from build123d import *

# Parameters (mm, degrees)
F0_R     = 8
F0_R_2   = 7
F1_DEPTH = 8.15
F2_DEPTH = 10
F3_DEPTH = 9
F5_W     = 115
F5_H     = 65
F6_DEPTH = 0.5
F8_DEPTH = 20
F11_R    = 1.5


# Not quite as in the source:
# - a fillet or chamfer that OpenCascade refuses, or shapes differently, is made with other operations: its cross-section is extruded or revolved along the edge and cut away or added


with BuildPart() as f1:
    # F0 (on Top) → F1 (new body)
    with BuildSketch(Plane.XY):
        with BuildLine():
            Line((-67.5, -39), (67.5, -39))
            ThreePointArc((67.5, -39), (71.7426406871, -37.2426406871), (73.5, -33))
            Line((73.5, -33), (73.5, 33))
            ThreePointArc((73.5, 33), (71.7426406871, 37.2426406871), (67.5, 39))
            Line((67.5, 39), (-67.5, 39))
            ThreePointArc((-67.5, 39), (-71.7426406871, 37.2426406871), (-73.5, 33))
            Line((-73.5, 33), (-73.5, -33))
            ThreePointArc((-73.5, -33), (-71.7426406871, -37.2426406871), (-67.5, -39))
        make_face()
        with Locations((-53.5, 0)):
            Circle(F0_R, mode=Mode.SUBTRACT)
        with Locations((-30.5, 0)):
            Circle(F0_R_2, mode=Mode.SUBTRACT)
        with Locations((-53.5, 0)):
            Circle(F0_R)
        with Locations((-30.5, 0)):
            Circle(F0_R_2)
    extrude(amount=F1_DEPTH)

    # F0 (on Top) → F2 (join)
    with BuildSketch(Plane.XY):
        with Locations((-53.5, 0)):
            Circle(F0_R)
    extrude(amount=F2_DEPTH)

    # F0 (on Top) → F3 (join)
    with BuildSketch(Plane.XY):
        with Locations((-30.5, 0)):
            Circle(F0_R_2)
    extrude(amount=F3_DEPTH)

    # F4: fillet of radius 4 on 1 edges, made by hand

    # F4_s1 → F4_t2 (revolve)
    with BuildSketch(Plane.XZ):
        with BuildLine():
            ThreePointArc((-42.1269450049, 8.15), (-44.0504834111, 8.6428644167), (-45.5, 10))
            Line((-45.5, 10), (-45.5, 8.15))
            Line((-45.5, 8.15), (-42.1269450049, 8.15))
        make_face()
    revolve(axis=Axis((-53.5, 0, 8.15), (0, 0, -1)))

    # F5 (on Top) → F6 (cut)
    with BuildSketch(Plane.XY):
        Rectangle(F5_W, F5_H)
    extrude(amount=F6_DEPTH, mode=Mode.SUBTRACT)

    # F7 (on face) → F8 (join)
    with BuildSketch(Plane.YZ.offset(73.5)):
        with BuildLine():
            ThreePointArc((7.4520160146, 3), (9.4520160146, 5), (7.4520160146, 7))
            Line((7.4520160146, 7), (-6.5479839854, 7))
            ThreePointArc((-6.5479839854, 7), (-8.5479839854, 5), (-6.5479839854, 3))
            Line((-6.5479839854, 3), (7.4520160146, 3))
        make_face()
        with BuildLine():
            ThreePointArc((-1.5, 5), (0, 6.5), (1.5, 5))
            ThreePointArc((1.5, 5), (0, 3.5), (-1.5, 5))
        make_face(mode=Mode.SUBTRACT)
        with BuildLine():
            Line((-1.5, 5), (1.5, 5))
            ThreePointArc((1.5, 5), (0, 6.5), (-1.5, 5))
        make_face()
        with BuildLine():
            ThreePointArc((-1.5, 5), (0, 3.5), (1.5, 5))
            Line((1.5, 5), (-1.5, 5))
        make_face()
    extrude(amount=F8_DEPTH)

    # F12: sweep along a path in F10
    with BuildLine(Plane(origin=(0, 0, 5), x_dir=(1, 0, 0), z_dir=(0, 0, -1))) as f12_path:
        ThreePointArc((93.5, 0), (108.8125986956, 5.7360841116), (116.8597106736, 19.970631121))
    # F11 (on face) → F12 (sweep)
    with BuildSketch(Plane.YZ.offset(93.5)):
        with Locations((0, 5)):
            Circle(F11_R)
    sweep(path=f12_path.line)


solid = f1.part
Geometry check sheet. Reference: the model listing, model coordinates, mm. A direction names the side the tool comes from. Round coordinates to 2 decimals unless told otherwise and drop trailing zeros. Loops run counter-clockwise (first coordinate to the right, second up) from the corner with the lowest first, then second, coordinate; pieces in that order, holes last. Notation, with made-up numbers: (81, -40) - (104, -40) arc R9 cw to (104, -23) - close; hole circle Ø9 at (-19, 9). An arc over 180 degrees is marked (long way). One line per question, with ' | ' between items. Start each with the question number.
1. Cross-section at D-D on x = 86.5. Record the cut outline in (y, z).
2. Cross-section at B-B on x = -30.5. Record the cut outline in (y, z), then the cut area to 3 significant figures.
3. Scan lines: line 1 (Z direction, x = -23, y = 9); line 2 (Z direction, x = 28.5, y = 33); line 3 (X direction, y = 1, z = 6.75). Record each from-to range of solid material in increasing order. Write a range as [from, to].
4. Cross-section at A-A on y = 22.5. Record the cut outline in (x, z), then the cut area to 3 significant figures.
5. Cross-section at C-C on x = 13.5. Record the cut outline in (y, z), then the cut area to 3 significant figures.
6. Tool access check on faces 5 (the face through (-1, 0, 0.5)), 6 (the face through (83, 0, 3)), 7 (the face through (83.36, -8.548, 5.044)), 8 (the face through (83, 1, 7)). Record the directions out of +Z, -Z, +X, -X, +Y, -Y that give a thin tool (end or side, any length) a straight path to the whole face; none if there is none.
7. Draft check along X on faces 1 (the face through (71.696, -37.289, 4.018)), 2 (the face through (83.36, 9.45, 4.96)), 3 (the face through (93.5, 0.3, 3.3)), 4 (the face through (-73.5, 0, 4)). Enter one of: released by +X, released by -X, zero draft, split by the parting line, or undercut.
8. Depth check by flat-ended pin: pin 1 (4 mm diameter, centred on y = -2, z = 3, fed in from +X); pin 2 (4 mm diameter, centred on x = -28, y = -1.5, fed in from +Z); pin 3 (6 mm diameter, centred on x = -9, y = 11, fed in from -Z). Enter the tip coordinate at first touch or a pass-through.
Taken from the geometry:
1) outline: (-6.55, 3) - (7.45, 3) arc R2 ccw to (7.45, 7) - (-6.55, 7) arc R2 ccw to start
2) outline: (-39, 0) - (-32.5, 0) - (-32.5, 0.5) - (32.5, 0.5) - (32.5, 0) - (39, 0) - (39, 8.15) - (7, 8.15) - (7, 9) - (-7, 9) - (-7, 8.15) - (-39, 8.15) - close | area: 615 mm²
3) line 1: [0.5, 8.15] | line 2: [0, 8.15] | line 3: [-73.5, 93.5]
4) outline: (-73.5, 0) - (-57.5, 0) - (-57.5, 0.5) - (57.5, 0.5) - (57.5, 0) - (73.5, 0) - (73.5, 8.15) - (-73.5, 8.15) - close | area: 1,140 mm²
5) outline: (-39, 0) - (-32.5, 0) - (-32.5, 0.5) - (32.5, 0.5) - (32.5, 0) - (39, 0) - (39, 8.15) - (-39, 8.15) - close | area: 603 mm²
6) face 5: -Z | face 6: -Z, +X, +Y, -Y | face 7: -Y | face 8: +Z, +X, +Y, -Y
7) face 1: released by +X | face 2: zero draft | face 3: undercut | face 4: released by -X
8) pin 1: x = 108.16 | pin 2: z = 9 | pin 3: z = 0.5
